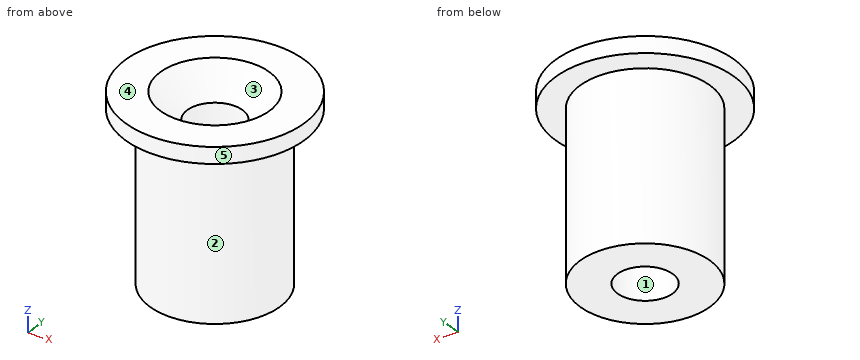
from build123d import *

# Parameters (mm, degrees)
REFRENTADO_PARA_TORNILLO_TAP_N_CON_CABEZ_D           = 3.4
REFRENTADO_PARA_TORNILLO_TAP_N_CON_CABEZ_CSINK_D     = 6.72
REFRENTADO_PARA_TORNILLO_TAP_N_CON_CABEZ_CSINK_ANGLE = 90


with BuildPart() as part:
    # Croquis1 → Revolución1 (revolve)
    with BuildSketch(Plane(origin=(0, 0, 0), x_dir=(1, 0, 0), z_dir=(0, 1, 0))):
        Polygon((-1.5, 11.25), (-1.5, 0), (-5.5, 0), (-5.5, 1), (-4, 1), (-4, 11.25), align=None)
    revolve(axis=Axis((0, 0, -19.14213198), (0, 0, 1)))

    # Refrentado para tornillo tapón con cabeza plana de clavija de M31 (through all)
    with Locations(Plane.XY):
        with Locations((0, 0)):
            CounterSinkHole(REFRENTADO_PARA_TORNILLO_TAP_N_CON_CABEZ_D / 2, REFRENTADO_PARA_TORNILLO_TAP_N_CON_CABEZ_CSINK_D / 2, counter_sink_angle=REFRENTADO_PARA_TORNILLO_TAP_N_CON_CABEZ_CSINK_ANGLE)


solid = part.part
The listing builds one solid part. Answer for the finished solid, in the listing's coordinates (mm). Face numbers are marked on the shaded views. A direction names the side the tool comes from. Coordinates: 2 decimals unless noted, no trailing zeros. Write each loop counter-clockwise with the first axis right and the second up, starting at its lowest first coordinate (ties: lowest second). Pieces come first, ordered by that corner, then holes. Notation, with made-up numbers: (63, 68.5) - (69, 68.5) arc R16 cw to (69, 93.5) - close; hole circle Ø8 at (-1, 58.25). An arc over 180 degrees is marked (long way). Put each result on its own line as item: value.
1. The part is cut by section A-A on y = 0. Give the vertices of the cut face in (x, z).
Answer sheet:
outline: (-5.5, -1) - (-4, -1) - (-4, -11.25) - (-1.7, -11.25) - (-1.7, -1.66) - (-3.36, 0) - (-5.5, 0) - close; (1.7, -11.25) - (4, -11.25) - (4, -1) - (5.5, -1) - (5.5, 0) - (3.36, 0) - (1.7, -1.66) - close
2. Determine the mould class of the marked faces 3, 4 and 5 for opening direction X: pulls with the +X half, pulls with the -X half, needs draft (parallel to the pull), parting line crosses it, or undercut.
Answer sheet:
face 3: undercut
face 4: needs draft
face 5: parting line crosses it
3. The part is cut by section C-C on z = -10.5. Give the vertices of the cut face in (x, y), plus the area to 3 significant figures.
Answer sheet:
outline: circle Ø8 at (0, 0); hole circle Ø3.4 at (0, 0)
area: 41.2 mm^2
4. Flat-ended cylindrical pins translate along their axes: pin 1 Ø5 at (y, z) = (-3.5, -4.5) entering from +X; pin 2 Ø1.5 at (x, y) = (4, -4) entering from +Z; pin 3 Ø1.5 at (y, z) = (-2, -5.5) entering from +X; pin 4 Ø3 at (x, y) = (0, 0) entering from +Z. Find the tip coordinate at first contact, or state that the pin passes through.
Answer sheet:
pin 1: stops at x = 3.87
pin 2: stops at z = 0
pin 3: stops at x = 3.8
pin 4: passes through
5. The part is cut by section D-D on x = 4.5. Give the vertices of the cut face in (y, z).
Answer sheet:
outline: (-3.16, -1) - (3.16, -1) - (3.16, 0) - (-3.16, 0) - close
6. A tool of negligible diameter and unlimited length cuts with its end or side. For the marked faces 1 and 2, from which of +Z, -Z, +X, -X, +Y, -Y can it reach the whole face along a straight path? Write none if from no direction.
Answer sheet:
face 1: +Z, -Z
face 2: -Z
7. Find the intervals of material crossed by line 1 along X through (y, z) = (0, -6.5); line 2 along Z through (x, y) = (-0.75, -4.25), in increasing order. Write a range as from..to.
Answer sheet:
line 1: x = -4..-1.7, 1.7..4
line 2: z = -1..0
